Input: part model. Units: mm. Frame: model coordinates. Face numbers are marked on the shaded views. A direction names the side the tool comes from. Round coordinates to 2 decimals unless told otherwise and drop trailing zeros. Order: outer loops, then holes, each group sorted by start corner. A loop starts at its lowest first (then second) coordinate and runs counter-clockwise, first axis right, second up. Notation, with made-up numbers: (28.5, 10.25) - (79.5, 10.25) arc R14 cw to (79.5, 20.25) - close; hole circle Ø3 at (21, 13.25). An arc over 180 degrees is marked (long way). One line per item, written item: value. Start each with the question number.
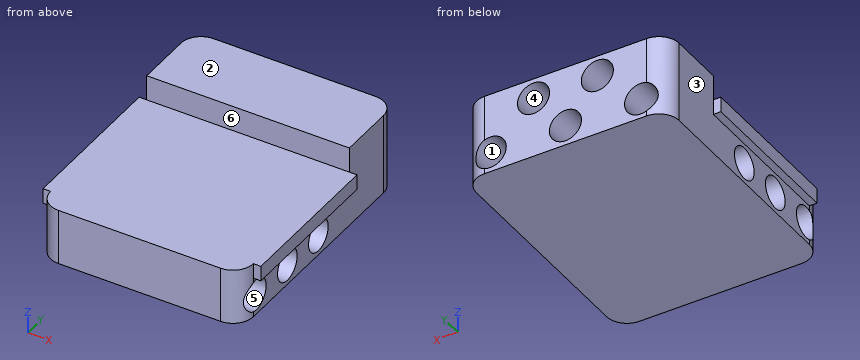
from build123d import *

# Parameters (mm, degrees)
F0_W         = 50.8
F0_H         = 38.1
F1_DEPTH     = 10.16
F2_R         = 4.01955
F3_DEPTH     = 23.495
F4_R         = 4.01955
F5_DEPTH     = 23.495
F6_DEPTH     = 25.4
F7_W         = 50.8
F7_H         = 19.05
F8_DEPTH     = 10.16
F9_R         = 4.01955
F10_DEPTH    = 15.24
F11_T1_DEPTH = 35.56
F12_T1_DEPTH = 45.72
F13_DEPTH    = 3.81
F15_W        = 39.37
F15_H        = 3.81
F16_DEPTH    = 1.905
F14_W        = 39.37
F14_H        = 3.81
F17_DEPTH    = 1.905


# Not quite as in the source:
# - a fillet or chamfer that OpenCascade refuses, or shapes differently, is made with other operations: its cross-section is extruded or revolved along the edge and cut away or added


with BuildPart() as f1:
    # F0 (on Top) → F1 (new body)
    with BuildSketch(Plane.XY):
        Rectangle(F0_W, F0_H)
    extrude(amount=F1_DEPTH)

    # F2 (on face) → F3 (cut)
    with BuildSketch(Plane(origin=(-25.4, 0, 0), x_dir=(0, -1, 0), z_dir=(-1, 0, 0))):
        with Locations((-12.7, 5.08)):
            Circle(F2_R)
        with Locations((0, 5.08)):
            Circle(F2_R)
        with Locations((12.7, 5.08)):
            Circle(F2_R)
    extrude(amount=-F3_DEPTH, mode=Mode.SUBTRACT)

    # F4 (on face) → F5 (cut)
    with BuildSketch(Plane.YZ.offset(25.4)):
        with Locations((-12.7, 5.08)):
            Circle(F4_R)
        with Locations((0, 5.08)):
            Circle(F4_R)
        with Locations((12.7, 5.08)):
            Circle(F4_R)
    extrude(amount=-F5_DEPTH, mode=Mode.SUBTRACT)

    # F6 (add): a face of the model
    f6_faces = [f1.faces().sort_by_distance(p)[0] for p in [
        (0, 19.05, 5.08),
    ]]
    extrude(f6_faces, amount=F6_DEPTH)

    # F7 (on face) → F8 (join)
    with BuildSketch(Plane.XY.offset(10.16)):
        with Locations((0, 34.925)):
            Rectangle(F7_W, F7_H)
    extrude(amount=F8_DEPTH)

    # F9 (on face) → F10 (cut)
    with BuildSketch(Plane(origin=(0, 44.45, 0), x_dir=(-1, 0, 0), z_dir=(0, 1, 0))):
        with Locations((0, 5.08)):
            Circle(F9_R)
        with Locations((-8.001, 15.24)):
            Circle(F9_R)
        with Locations((-18.84045, 5.08)):
            Circle(F9_R)
        with Locations((8.001, 15.24)):
            Circle(F9_R)
        with Locations((18.84045, 5.08)):
            Circle(F9_R)
    extrude(amount=-F10_DEPTH, mode=Mode.SUBTRACT)

    # F11: fillet of radius 5.08 on 2 edges, made by hand

    # F11_s2 → F11_t1 (cut)
    with BuildSketch(Plane.XY.offset(-12.7)):
        with BuildLine():
            ThreePointArc((-20.32, -19.05), (-23.9121024484, -17.5621024484), (-25.4, -13.97))
            Line((-25.4, -13.97), (-25.4, -19.05))
            Line((-25.4, -19.05), (-20.32, -19.05))
        make_face()
        with BuildLine():
            ThreePointArc((20.32, -19.05), (23.9121024484, -17.5621024484), (25.4, -13.97))
            Line((25.4, -13.97), (25.4, -19.05))
            Line((25.4, -19.05), (20.32, -19.05))
        make_face()
    extrude(amount=F11_T1_DEPTH, mode=Mode.SUBTRACT)

    # F12: fillet of radius 5.08 on 2 edges, made by hand

    # F12_s2 → F12_t1 (cut)
    with BuildSketch(Plane.XY.offset(-12.7)):
        with BuildLine():
            ThreePointArc((-25.4, 39.37), (-23.9121024484, 42.9621024484), (-20.32, 44.45))
            Line((-20.32, 44.45), (-25.4, 44.45))
            Line((-25.4, 44.45), (-25.4, 39.37))
        make_face()
        with BuildLine():
            ThreePointArc((20.32, 44.45), (23.9121024484, 42.9621024484), (25.4, 39.37))
            Line((25.4, 39.37), (25.4, 44.45))
            Line((25.4, 44.45), (20.32, 44.45))
        make_face()
    extrude(amount=F12_T1_DEPTH, mode=Mode.SUBTRACT)

    # F13 (add): a face of the model
    f13_faces = [f1.faces().sort_by_distance(p)[0] for p in [
        (0, 3.2789617265, 10.16),
    ]]
    extrude(f13_faces, amount=F13_DEPTH)

    # F15 (on face) → F16 (join)
    with BuildSketch(Plane(origin=(-25.4, 0, 0), x_dir=(0, -1, 0), z_dir=(-1, 0, 0))):
        with Locations((-5.715, 12.065)):
            Rectangle(F15_W, F15_H)
    extrude(amount=F16_DEPTH)

    # F14 (on face) → F17 (join)
    with BuildSketch(Plane.YZ.offset(25.4)):
        with Locations((5.715, 12.065)):
            Rectangle(F14_W, F14_H)
    extrude(amount=F17_DEPTH)


solid = f1.part
1. Section A-A (x = 0). Return the cut outline in (y, z), then the cut area to 3 significant figures.
2. Set-up query: the marked faces 4, 5 and 6. Return all of +Z, -Z, +X, -X, +Y, -Y with unobstructed straight access to the full face (end or side cutting, diameter ignored); none if empty.
3. Line query: line 1 (Z direction, x = 20.75, y = 12.7); line 2 (Y direction, x = 21.5, z = 5.75); line 3 (X direction, y = 39, z = 13.25). Output: solid intervals per line, ascending. Write a range as from..to.
4. Pull-direction query (Z, two-part tool) for the marked faces 1, 2 and 3; classes: released by +Z, released by -Z, zero draft, split by the parting line, or undercut.
5. Section B-B (z = 15.24). Return the cut outline in (x, y).
6. Section D-D (x = 5.5). Return the cut outline in (y, z), then the cut area to 3 significant figures.
7. Section C-C (y = -6). Return the cut outline in (x, z) (3 decimals), then the cut area to 3 significant figures.
8. Pin query (flat end, axial travel): pin 1 (6.5 mm diameter, centred on y = -14.5, z = 6, fed in from -X); pin 2 (4 mm diameter, centred on y = 12.5, z = 4, fed in from -X) (3 decimals); pin 3 (6 mm diameter, centred on x = 20, y = 13.5, fed in from +Z). Return the tip coordinate at first contact, or that it passes through.
Solved:
1. outline: (-19.05, 0) - (44.45, 0) - (44.45, 1.06) - (29.21, 1.06) - (29.21, 9.1) - (44.45, 9.1) - (44.45, 20.32) - (25.4, 20.32) - (25.4, 13.97) - (-19.05, 13.97) - close
1. area: 886 mm²
2. face 4: +Y
2. face 5: +X
2. face 6: +Z, +X, -X, -Y
3. line 1: z = 0..1.06, 9.1..13.97
3. line 2: y = -18.91..-16.66, -8.74..-3.96, 3.96..8.74, 16.66..29.21
3. line 3: x = -25.4..-11.49, -4.51..4.51, 11.49..25.4
4. face 1: undercut
4. face 2: released by +Z
4. face 3: zero draft
5. outline: (-25.4, 25.4) - (25.4, 25.4) - (25.4, 39.37) arc R5.08 ccw to (20.32, 44.45) - (12.02, 44.45) - (12.02, 29.21) - (3.98, 29.21) - (3.98, 44.45) - (-3.98, 44.45) - (-3.98, 29.21) - (-12.02, 29.21) - (-12.02, 44.45) - (-20.32, 44.45) arc R5.08 ccw to (-25.4, 39.37) - close
6. outline: (-19.05, 0) - (44.45, 0) - (44.45, 12.09) - (29.21, 12.09) - (29.21, 18.39) - (44.45, 18.39) - (44.45, 20.32) - (25.4, 20.32) - (25.4, 13.97) - (-19.05, 13.97) - close; hole circle Ø8.04 at (-12.7, 5.08); hole circle Ø8.04 at (0, 5.08); hole circle Ø8.04 at (12.7, 5.08)
6. area: 760 mm²
7. outline: (-27.305, 10.16) - (-25.4, 10.16) - (-25.4, 0) - (25.4, 0) - (25.4, 10.16) - (27.305, 10.16) - (27.305, 13.97) - (-27.305, 13.97) - close
7. area: 724 mm²
8. pin 1: stops at x = -25.4
8. pin 2: stops at x = -1.905
8. pin 3: stops at z = 13.97
